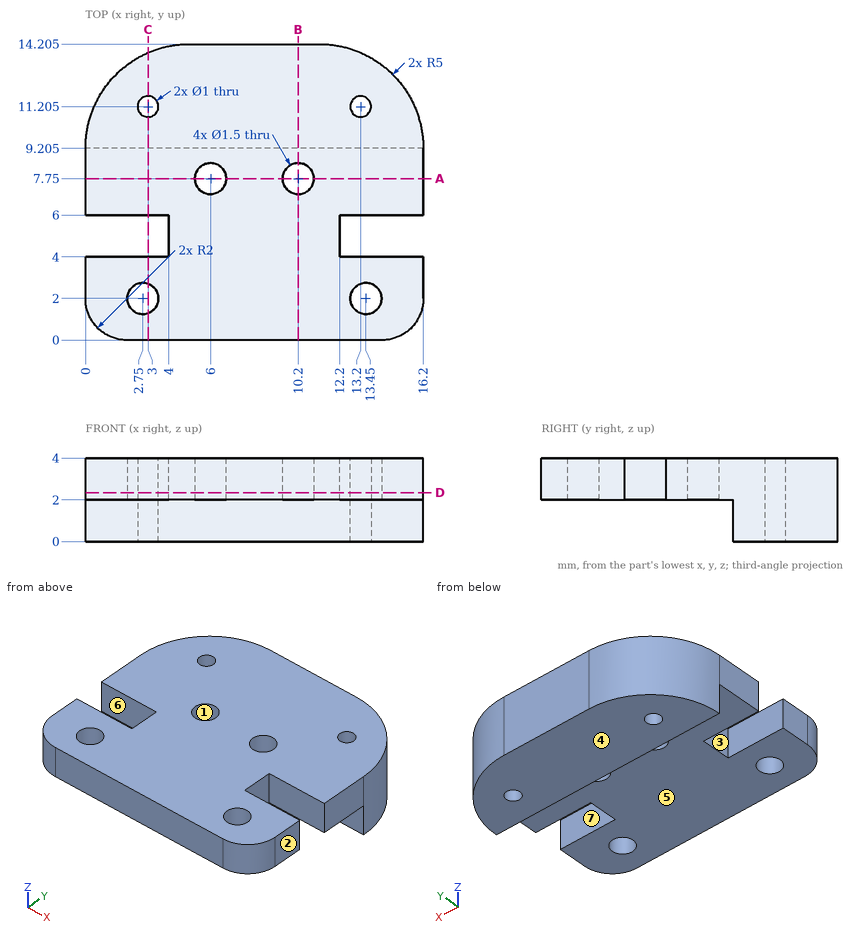
The drawing under review shows one solid part. Ordinate dimensions are in mm from its lowest x, y, z. A direction names the side the tool comes from. Coordinates: 2 decimals unless noted, no trailing zeros. Loops run counter-clockwise (first coordinate to the right, second up) from the corner with the lowest first, then second, coordinate; pieces in that order, holes last. Notation, with made-up numbers: (36, -10.75) -> (95, -10.75) arc R28 cw to (95, 23.25) -> close; hole circle Ø11 at (39, 53). An arc over 180 degrees is marked (long way). Answer as a JSON object with one key per item and string values.
Q1. Take a section at A-A on y = 7.75. Give the boundary of the cut face in (x, z).
Answer block:
{"outline": "(0, 2) -> (5.25, 2) -> (5.25, 4) -> (0, 4) -> close; (6.75, 2) -> (9.45, 2) -> (9.45, 4) -> (6.75, 4) -> close; (10.95, 2) -> (16.2, 2) -> (16.2, 4) -> (10.95, 4) -> close"}
Q2. Take a section at B-B on x = 10.2. Give the boundary of the cut face in (y, z) (3 decimals).
Answer block:
{"outline": "(0, 2) -> (7, 2) -> (7, 4) -> (0, 4) -> close; (8.5, 2) -> (9.205, 2) -> (9.205, 0) -> (14.205, 0) -> (14.205, 4) -> (8.5, 4) -> close"}
Q3. The part is to be moulded in two halves that separate along X. For the marked faces 1, 2 and 3, say which applies: +X half, -X half, draft (parallel to the pull), parting line (faces both ways), or undercut.
Answer block:
{"face 1": "undercut", "face 2": "+X half", "face 3": "-X half"}
Q4. Tool access review of the marked faces 4, 5, 6 and 7: name each direction out of +Z, -Z, +X, -X, +Y, -Y from which nothing blocks a thin tool from reaching the whole face with its end or side.
Answer block:
{"face 4": "-Z, +X, -X, +Y, -Y", "face 5": "-Z, +X, -X, -Y", "face 6": "+Z, -Z, -X", "face 7": "+Z, -Z, +X"}
Q5. Clearance check with flat-ended pins moving along their axes: pin 1 Ø1 at (x, z) = (1, 3) entering from +Y; pin 2 Ø1 at (x, z) = (14.5, 2.5) entering from +Y; pin 3 Ø1.7 at (x, y) = (10.2, 7.75) entering from -Z; pin 4 Ø1.4 at (x, y) = (6, 7.75) entering from -Z (1 decimal). State where each tip first meets the part, or that it passes through.
Answer block:
{"pin 1": "stops at y = 12.78", "pin 2": "stops at y = 13.35", "pin 3": "stops at z = 2", "pin 4": "passes through"}
Q6. Take a section at C-C on x = 3. Give the boundary of the cut face in (y, z) (3 decimals).
Answer block:
{"outline": "(0, 2) -> (1.293, 2) -> (1.293, 4) -> (0, 4) -> close; (2.707, 2) -> (4, 2) -> (4, 4) -> (2.707, 4) -> close; (6, 2) -> (9.205, 2) -> (9.205, 0) -> (10.705, 0) -> (10.705, 4) -> (6, 4) -> close; (11.705, 0) -> (13.788, 0) -> (13.788, 4) -> (11.705, 4) -> close"}
Q7. Take a section at D-D on z = 2.35. Give the boundary of the cut face in (x, y) (3 decimals), plus the area to 3 significant figures.
Answer block:
{"outline": "(0, 2) arc R2 ccw to (2, 0) -> (14.2, 0) arc R2 ccw to (16.2, 2) -> (16.2, 4) -> (12.2, 4) -> (12.2, 6) -> (16.2, 6) -> (16.2, 9.205) arc R5 ccw to (11.2, 14.205) -> (5, 14.205) arc R5 ccw to (0, 9.205) -> (0, 6) -> (4, 6) -> (4, 4) -> (0, 4) -> close; hole circle Ø1.5 at (2.75, 2); hole circle Ø1 at (3, 11.205); hole circle Ø1.5 at (6, 7.75); hole circle Ø1.5 at (10.2, 7.75); hole circle Ø1.5 at (13.45, 2); hole circle Ø1 at (13.2, 11.205)", "area": "193 mm^2"}
Q8. To check wall thickness, follow L1, parallel to X at y = 7.75, z = 2.75; L2, parallel to X at y = 2, z = 3.2; L3, parallel to Y at x = 2.75, z = 2.5. State the ranges of each line that lie inside material, in increasing order.
Answer block:
{"L1": "x = 0 to 5.25, 6.75 to 9.45, 10.95 to 16.2", "L2": "x = 0 to 2, 3.5 to 12.7, 14.2 to 16.2", "L3": "y = 0 to 1.25, 2.75 to 4, 6 to 10.77, 11.64 to 13.67"}
